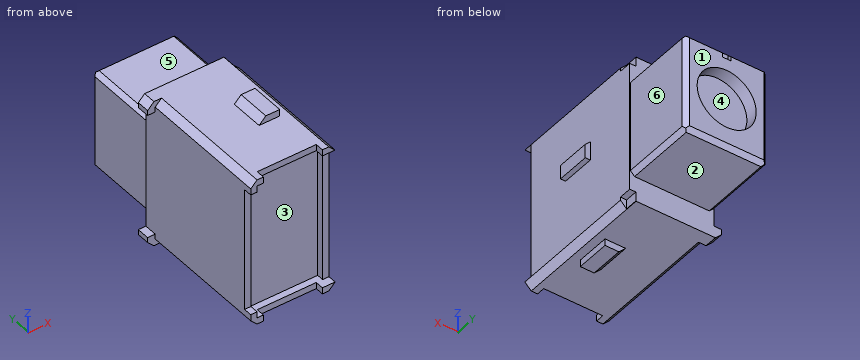
Autodesk Inventor part; units mm, degrees
ref_plane "to_bracket_r_XY" through (-2.54, -4.3078, 0) normal (1, 0, 0) x (0, 0, -1)
ref_plane "to_bracket_r_YZ" through (-2.54, -4.3078, 0) normal (0, 0, -1) x (0, 1, 0)
ref_plane "to_bracket_r_ZX" through (-2.54, -4.3078, 0) normal (0, 1, 0) x (1, 0, 0)
sketch "Sketch_1" plane through (0, 0, 0) normal (0, 1, 0) x (-1, 0, 0)
  line L0 (2.54, -4.1148) -> (2.54, 4.1148)
  line L1 (2.54, 4.1148) -> (2.159, 4.4958)
  line L2 (2.159, 4.4958) -> (-2.159, 4.4958)
  line L3 (-2.159, 4.4958) -> (-2.54, 4.1148)
  line L4 (-2.54, 4.1148) -> (-2.54, -4.1148)
  line L5 (-2.54, -4.1148) -> (-2.159, -4.4958)
  line L6 (-2.159, -4.4958) -> (2.159, -4.4958)
  line L7 (2.159, -4.4958) -> (2.54, -4.1148)
extrude "Extrusion1" add sketch "Sketch_1" against normal blind 8.6106
sketch "Sketch_2" plane through (0, -8.6106, 0) normal (0, 1, 0) x (1, 0, 0)
  line L0 (-2.54, 3.7338) -> (-2.54, -3.7338)
  line L1 (-2.54, -3.7338) -> (-2.159, -3.7338)
  line L2 (-2.159, -3.7338) -> (-2.159, -4.1148)
  line L3 (-2.159, -4.1148) -> (-1.778, -4.1148)
  line L4 (-1.778, -4.1148) -> (-1.778, -4.4958)
  line L5 (-1.778, -4.4958) -> (1.778, -4.4958)
  line L6 (1.778, -4.4958) -> (1.778, -4.1148)
  line L7 (1.778, -4.1148) -> (2.54, -4.1148)
  line L8 (2.54, -4.1148) -> (2.54, 4.1148)
  line L9 (2.54, 4.1148) -> (1.778, 4.1148)
  line L10 (1.778, 4.1148) -> (1.778, 4.4958)
  line L11 (1.778, 4.4958) -> (-1.778, 4.4958)
  line L12 (-1.778, 4.4958) -> (-1.778, 4.1148)
  line L13 (-1.778, 4.1148) -> (-2.159, 4.1148)
  line L14 (-2.159, 4.1148) -> (-2.159, 3.7338)
  line L15 (-2.159, 3.7338) -> (-2.54, 3.7338)
extrude "Extrusion2" cut sketch "Sketch_2" along normal blind 0.508
sketch "Sketch_21" plane through (0, -8.6106, 0) normal (0, 1, 0) x (1, 0, 0)
  line L0 (-2.159, -4.1148) -> (2.159, -4.1148)
  line L1 (2.159, -4.1148) -> (2.159, 4.1148)
  line L2 (2.159, 4.1148) -> (-2.159, 4.1148)
  line L3 (-2.159, 4.1148) -> (-2.159, -4.1148)
extrude "Extrusion3" cut sketch "Sketch_21" along normal blind 0.9144
sketch "Sketch_3" plane through (0, 0, 0) normal (0, 1, 0) x (-1, 0, 0)
  line L0 (-2.1717, -3.9243) -> (-2.6162, -3.9243)
  line L1 (-2.6162, -3.9243) -> (-2.6162, 3.9243)
  line L2 (-2.6162, 3.9243) -> (-2.1717, 3.9243)
  line L3 (-2.1717, 3.9243) -> (-2.1717, 4.4958)
  line L4 (-2.1717, 4.4958) -> (-2.921, 4.4958)
  line L5 (-2.921, 4.4958) -> (-2.921, -4.4958)
  line L6 (-2.921, -4.4958) -> (-2.1717, -4.4958)
  line L7 (-2.1717, -4.4958) -> (-2.1717, -3.9243)
extrude "Extrusion4" cut sketch "Sketch_3" against normal blind 0.762
sketch "Sketch_4" plane through (0, 0, 0) normal (0, 1, 0) x (-1, 0, 0)
  line L0 (2.9972, -3.81) -> (2.5019, -3.81)
  line L1 (2.5019, -3.81) -> (2.5019, 3.81)
  line L2 (2.5019, 3.81) -> (2.9972, 3.81)
  line L3 (2.9972, 3.81) -> (2.9972, 4.1148)
  line L4 (2.9972, 4.1148) -> (2.6162, 4.4958)
  line L5 (2.6162, 4.4958) -> (0.0762, 4.4958)
  line L6 (0.0762, 4.4958) -> (0.0762, -4.4958)
  line L7 (0.0762, -4.4958) -> (2.6162, -4.4958)
  line L8 (2.6162, -4.4958) -> (2.9972, -4.1148)
  line L9 (2.9972, -4.1148) -> (2.9972, -3.81)
extrude "Extrusion5" add sketch "Sketch_4" against normal blind 0.762
sketch "Sketch_5" plane through (0, -3.241, 0) normal (0, 1, 0) x (1, 0, 0)
  line L0 (0.41, -4.4958) -> (0.8164, -4.9022)
  line L1 (0.8164, -4.9022) -> (1.651, -4.9022)
  line L2 (1.651, -4.9022) -> (1.651, -4.4958)
  line L3 (1.651, -4.4958) -> (0.41, -4.4958)
extrude "Extrusion6" add sketch "Sketch_5" against normal blind 2.032
sketch "Sketch_6" plane through (0, -3.241, 0) normal (0, 1, 0) x (1, 0, 0)
  line L0 (0.41, 4.4958) -> (1.651, 4.4958)
  line L1 (1.651, 4.4958) -> (1.651, 4.9022)
  line L2 (1.651, 4.9022) -> (0.8164, 4.9022)
  line L3 (0.8164, 4.9022) -> (0.41, 4.4958)
extrude "Extrusion7" add sketch "Sketch_6" against normal blind 2.032
sketch "Sketch_7" plane through (0, -3.241, 0) normal (0, 1, 0) x (1, 0, 0)
  line L0 (2.54, 0) -> (2.54, -1.1394)
  line L1 (2.54, -1.1394) -> (2.8448, -0.8346)
  line L2 (2.8448, -0.8346) -> (2.8448, 0)
  line L3 (2.8448, 0) -> (2.54, 0)
extrude "Extrusion8" add sketch "Sketch_7" against normal blind 2.032
sketch "Sketch_8" plane through (0, 0, 0) normal (0, 1, 0) x (-1, 0, 0)
  line L0 (2.5019, -2.7432) -> (2.5019, 2.7432)
  line L1 (2.5019, 2.7432) -> (2.2479, 2.9972)
  line L2 (2.2479, 2.9972) -> (-2.2479, 2.9972)
  line L3 (-2.2479, 2.9972) -> (-2.5019, 2.7432)
  line L4 (-2.5019, 2.7432) -> (-2.5019, -2.7432)
  line L5 (-2.5019, -2.7432) -> (-2.2479, -2.9972)
  line L6 (-2.2479, -2.9972) -> (2.2479, -2.9972)
  line L7 (2.2479, -2.9972) -> (2.5019, -2.7432)
extrude "Extrusion9" add sketch "Sketch_8" along normal blind 4.4958
sketch "Sketch_9" plane through (0, 0, 0) normal (1, 0, 0) x (0, 1, 0)
  line L0 (0, 3.2953) -> (0, 2.9972)
  line L1 (0, 2.9972) -> (4.2418, 2.9972)
  line L2 (4.2418, 2.9972) -> (4.4958, 2.7432)
  line L3 (4.4958, 2.7432) -> (4.4958, -2.7432)
  line L4 (4.4958, -2.7432) -> (4.2418, -2.9972)
  line L5 (4.2418, -2.9972) -> (0, -2.9972)
  line L6 (0, -2.9972) -> (0, -3.2953)
  line L7 (0, -3.2953) -> (4.5957, -3.2953)
  line L8 (4.5957, -3.2953) -> (4.5957, 3.2953)
  line L9 (4.5957, 3.2953) -> (0, 3.2953)
extrude "Extrusion10" cut sketch "Sketch_9" along normal mid plane 5.0038
sketch "Sketch_10" plane through (0, 0, 0) normal (0, 0, 1) x (1, 0, 0)
  line L0 (-3.2953, 0) -> (-2.5019, 0)
  line L1 (-2.5019, 0) -> (-2.5019, 4.2418)
  line L2 (-2.5019, 4.2418) -> (-2.2479, 4.4958)
  line L3 (-2.2479, 4.4958) -> (2.2479, 4.4958)
  line L4 (2.2479, 4.4958) -> (2.5019, 4.2418)
  line L5 (2.5019, 4.2418) -> (2.5019, 0)
  line L6 (2.5019, 0) -> (3.2953, 0)
  line L7 (3.2953, 0) -> (3.2953, 4.5957)
  line L8 (3.2953, 4.5957) -> (-3.2953, 4.5957)
  line L9 (-3.2953, 4.5957) -> (-3.2953, 0)
extrude "Extrusion11" cut sketch "Sketch_10" along normal mid plane 5.9944
sketch "Sketch12" plane through (0, 4.4958, 0) normal (0, 1, 0) x (1, 0, 0)
  point P0 (0, 0)
hole "Drilling 1" at (0, 4.4958, 0) direction (0, -1, 0) diameter 3.556 depth 0.762
sketch "Sketch_28" plane through (0, 4.4958, 0) normal (0, 1, 0) x (1, 0, 0)
  line L0 (-0.254, -2.4892) -> (-0.254, -2.9972)
  line L1 (-0.254, -2.9972) -> (0.254, -2.9972)
  line L2 (0.254, -2.9972) -> (0.254, -2.4892)
  line L3 (0.254, -2.4892) -> (-0.254, -2.4892)
extrude "Extrusion12" cut sketch "Sketch_28" against normal blind 0.254
ref_plane "to_bracket_r_XY" through (-2.54, -4.3078, 0) normal (1, 0, 0) x (0, 0, -1)
ref_plane "to_bracket_r_YZ" through (-2.54, -4.3078, 0) normal (0, 0, -1) x (0, 1, 0)
ref_plane "to_bracket_r_ZX" through (-2.54, -4.3078, 0) normal (0, 1, 0) x (1, 0, 0)
ref_plane "to_bracket_r2_XY" through (-4.3942, -4.318, 0) normal (1, 0, 0) x (0, 0, -1)
ref_plane "to_bracket_r2_YZ" through (-4.3942, -4.318, 0) normal (0, 0, -1) x (0, 1, 0)
ref_plane "to_bracket_r2_ZX" through (-4.3942, -4.318, 0) normal (0, 1, 0) x (1, 0, 0)
ref_plane "to_bracket_s_XY" through (-2.54, -4.7015, 0) normal (1, 0, 0) x (0, 0, -1)
ref_plane "to_bracket_s_YZ" through (-2.54, -4.7015, 0) normal (0, 0, -1) x (0, 1, 0)
ref_plane "to_bracket_s_ZX" through (-2.54, -4.7015, 0) normal (0, 1, 0) x (1, 0, 0)
ref_plane "to_bracket_s2_XY" through (-4.3942, -4.7142, 0) normal (1, 0, 0) x (0, 0, -1)
ref_plane "to_bracket_s2_YZ" through (-4.3942, -4.7142, 0) normal (0, 0, -1) x (0, 1, 0)
ref_plane "to_bracket_s2_ZX" through (-4.3942, -4.7142, 0) normal (0, 1, 0) x (1, 0, 0)
ref_plane "to_bracket_v_XY" through (0, -4.1554, 4.3942) normal (0, 0, -1) x (1, 0, 0)
ref_plane "to_bracket_v_YZ" through (0, -4.1554, 4.3942) normal (1, 0, 0) x (0, -1, 0)
ref_plane "to_bracket_v_ZX" through (0, -4.1554, 4.3942) normal (0, -1, 0) x (0, 0, -1)
ref_plane "to_dummy_XY" through (0, 0, 0) normal (0, -1, 0) x (1, 0, 0)
ref_plane "to_dummy_YZ" through (0, 0, 0) normal (1, 0, 0) x (0, 0, 1)
ref_plane "to_dummy_ZX" through (0, 0, 0) normal (0, 0, 1) x (0, -1, 0)
ref_plane "to_terminal_XY" through (0, -7.3406, 0) normal (0, 1, 0) x (1, 0, 0)
ref_plane "to_terminal_YZ" through (0, -7.3406, 0) normal (1, 0, 0) x (0, 0, -1)
ref_plane "to_terminal_ZX" through (0, -7.3406, 0) normal (0, 0, -1) x (0, 1, 0)
ref_plane "to_toggle_XY" through (0, 4.4958, 0) normal (0, -1, 0) x (1, 0, 0)
ref_plane "to_toggle_YZ" through (0, 4.4958, 0) normal (1, 0, 0) x (0, 0, 1)
ref_plane "to_toggle_ZX" through (0, 4.4958, 0) normal (0, 0, 1) x (0, -1, 0)
properties part number "A1-toggle-body"
Read the model definition and answer for the solid it produces. Units are mm, in the model's axes. Face numbers are marked on the shaded views. A direction names the side the tool comes from. Coordinates: 2 decimals unless noted, no trailing zeros. Write each loop counter-clockwise with the first axis right and the second up, starting at its lowest first coordinate (ties: lowest second). Pieces come first, ordered by that corner, then holes. Notation, with made-up numbers: (50, 66) - (67, 66) arc R30 ccw to (67, 98) - close; hole circle Ø10 at (70, 2). An arc over 180 degrees is marked (long way). Answer as a JSON object with one key per item and string values. Group by question number.
1. A cutting plane is placed at A-A (y = 0.75). Determine the outline of the cut face in (x, z).
2. The mould has two halves that part along Z. Classify the marked faces 1, 2 and 3: +Z half, -Z half, draft (parallel to the pull), parting line (faces both ways), or undercut.
3. A cutting plane is placed at B-B (z = -3.5). Determine the outline of the cut face in (x, y).
4. Consider L1, parallel to X at y = 4.1, z = 0; L2, parallel to Z at x = 0, y = 4.2; L3, parallel to Y at x = -1.4, z = -3.25. Determine where each line is inside the solid, lowest interval first. Write a range as [from, to].
5. Which of the six approach directions +Z, -Z, +X, -X, +Y, -Y give full straight-line access (tool end or side, diameter ignored) to the marked faces 4, 5 and 6?
6. Each of these flat-tipped pins is pushed along its axis until it touches: P1, Ø1, axis at y = 2, z = 2, coming from the -X side; P2, Ø1, axis at y = -5.5, z = -2, coming from the +X side; P3, Ø1.5, axis at x = -2.5, y = -7, coming from the +Z side; P4, Ø0.5, axis at x = -1, y = -8.5, coming from the +Z side. Where does it stop, or does it pass through?
7. A cutting plane is placed at C-C (x = 0). Determine the outline of the cut face in (y, z), plus the area to 3 significant figures.
Worked out:
{
 "1": {"outline": "(-2.5, -2.74) - (-2.25, -3) - (2.25, -3) - (2.5, -2.74) - (2.5, 2.74) - (2.25, 3) - (-2.25, 3) - (-2.5, 2.74) - close"},
 "2": {"face 1": "draft", "face 2": "-Z half", "face 3": "undercut"},
 "3": {"outline": "(-2.54, -8.1) - (-2.16, -8.1) - (-2.16, -7.7) - (2.16, -7.7) - (2.16, -8.1) - (2.54, -8.1) - (2.54, 0) - (-2.54, 0) - close"},
 "4": {"L1": "x = [-2.5, -1.78], [1.78, 2.5]", "L2": "z = [-3, -1.78], [1.78, 3]", "L3": "y = [-7.7, 0]"},
 "5": {"face 4": "+Y", "face 5": "+Z, +X, -X, +Y", "face 6": "+Z, -Z, +X, +Y"},
 "6": {"P1": "stops at x = -2.5", "P2": "stops at x = 2.54", "P3": "stops at z = 4.5", "P4": "passes through"},
 "7": {"outline": "(-8.1, -4.5) - (0, -4.5) - (0, -3) - (4.24, -3) - (4.5, -2.74) - (4.5, -1.78) - (3.73, -1.78) - (3.73, 1.78) - (4.5, 1.78) - (4.5, 2.49) - (4.24, 2.49) - (4.24, 3) - (0, 3) - (0, 4.5) - (-8.1, 4.5) - (-8.1, 4.11) - (-7.7, 4.11) - (-7.7, -4.11) - (-8.1, -4.11) - close", "area": "93.6 mm²"}
}
